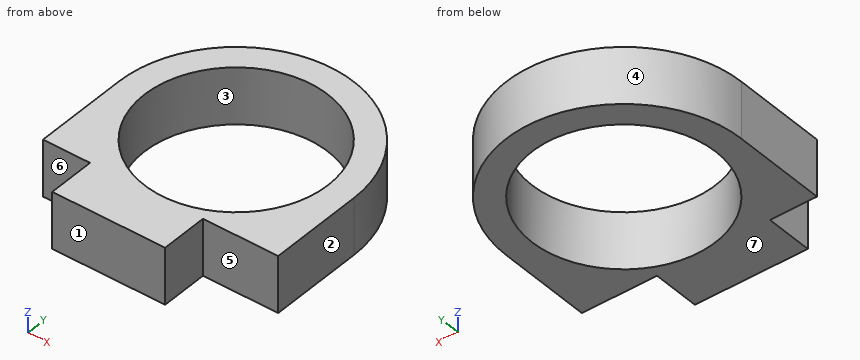
```python
from build123d import *

# Parameters (mm, degrees)
CROQUIS1_R              = 9.75
SALIENTE_EXTRUIR1_DEPTH = 6


with BuildPart() as part:
    # Croquis1 → Saliente-Extruir1 (new body)
    with BuildSketch(Plane.XY):
        with BuildLine():
            ThreePointArc((12.5, 0), (0, 12.5), (-12.5, 0))
            Line((-12.5, 0), (-12.5, -10))
            Line((-12.5, -10), (-7.5, -10))
            Line((-7.5, -10), (-7.5, -15))
            Line((-7.5, -15), (4.5, -15))
            Line((4.5, -15), (4.5, -10))
            Line((4.5, -10), (12.5, -10))
            Line((12.5, -10), (12.5, 0))
        make_face()
        Circle(CROQUIS1_R, mode=Mode.SUBTRACT)
    extrude(amount=SALIENTE_EXTRUIR1_DEPTH)


solid = part.part
```
Geometry check sheet. Reference: the model listing, model coordinates, mm. Face numbers are marked on the shaded views. A direction names the side the tool comes from. Round coordinates to 2 decimals unless told otherwise and drop trailing zeros. Order: outer loops, then holes, each group sorted by start corner. A loop starts at its lowest first (then second) coordinate and runs counter-clockwise, first axis right, second up. Notation, with made-up numbers: (45.5, 36.5) -> (60.5, 36.5) arc R19 ccw to (60.5, 65.5) -> close; hole circle Ø10 at (81.5, 45). An arc over 180 degrees is marked (long way). Return JSON: item names as keys, results as strings. Group by question number.
Q1. Section check B-B, the plane x = 0. Record the boundary of the cut face in (y, z), plus the area to 3 significant figures.
Q2. Gauge pin test, flat ends, axial feed: pin 1 (6 mm diameter, centred on x = 5, y = -0.5, fed in from -Z); pin 2 (2.5 mm diameter, centred on y = -11.5, z = 1.5, fed in from -X). Record the tip position at first contact, or that the pin passes through.
Q3. Release check for a two-part mould opening along Y. For the marked faces 1, 2, 3 and 4 record: released by +Y, released by -Y, zero draft, split by the parting line, or undercut.
Q4. Material ranges on probe 1 along Y at (x, z) = (0, 2.1); probe 2 along Y at (x, z) = (-3, 0.3); probe 3 along X at (y, z) = (-12.25, 3.45), recorded low to high. Write a range as from..to.
Q5. Section check A-A, the plane y = -9. Record the boundary of the cut face in (x, z), plus the area to 3 significant figures.
Q6. Section check C-C, the plane z = 3.85. Record the boundary of the cut face in (x, y).
Q7. Tool access check on the marked faces 5, 6 and 7. Record the directions out of +Z, -Z, +X, -X, +Y, -Y that give a thin tool (end or side, any length) a straight path to the whole face; none if there is none.
Numbers:
{
 "1": {"outline": "(-15, 0) -> (-9.75, 0) -> (-9.75, 6) -> (-15, 6) -> close; (9.75, 0) -> (12.5, 0) -> (12.5, 6) -> (9.75, 6) -> close", "area": "48.0 mm^2"},
 "2": {"pin 1": "through", "pin 2": "x = -7.5"},
 "3": {"face 1": "released by -Y", "face 2": "zero draft", "face 3": "undercut", "face 4": "released by +Y"},
 "4": {"probe 1": "-15..-9.75, 9.75..12.5", "probe 2": "-15..-9.28, 9.28..12.13", "probe 3": "-7.5..4.5"},
 "5": {"outline": "(-12.5, 0) -> (-3.75, 0) -> (-3.75, 6) -> (-12.5, 6) -> close; (3.75, 0) -> (12.5, 0) -> (12.5, 6) -> (3.75, 6) -> close", "area": "105 mm^2"},
 "6": {"outline": "(-12.5, -10) -> (-7.5, -10) -> (-7.5, -15) -> (4.5, -15) -> (4.5, -10) -> (12.5, -10) -> (12.5, 0) arc R12.5 ccw to (-12.5, 0) -> close; hole circle Ø19.5 at (0, 0)"},
 "7": {"face 5": "+Z, -Z, +X, -Y", "face 6": "+Z, -Z, -X, -Y", "face 7": "-Z, +X, -X, +Y, -Y"}
}
